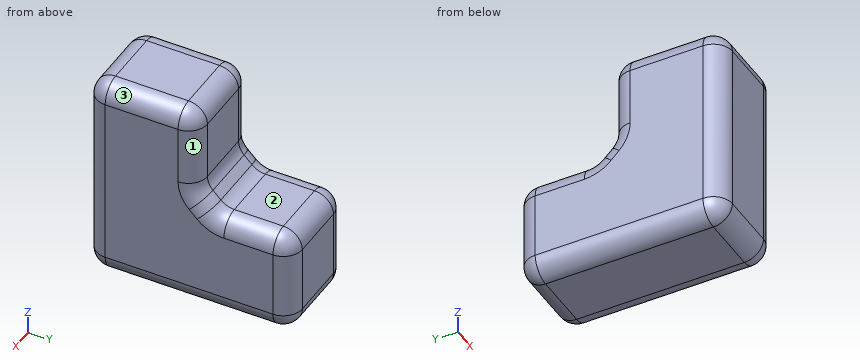
```python
from build123d import *

# Parameters (mm, degrees)
F0_W     = 25.4
F0_H     = 27.94
F1_DEPTH = 25.4
F2_SIZE  = 5.08
F3_F1_R  = 5.08
F3_F2_R  = 5.08


with BuildPart() as f1:
    # F0 (on Right) → F1 (new body)
    with BuildSketch(Plane.YZ):
        Polygon((-14.8341231188, -27.94), (14.8341231188, -27.94), (14.8341231188, 0), (14.8341231188, 27.94), (-14.8341231188, 27.94), align=None)
        with Locations((27.5341231188, -13.97)):
            Rectangle(F0_W, F0_H)
    extrude(amount=F1_DEPTH)

    # F2
    f2_edges = [f1.edges().sort_by_distance(p)[0] for p in [
        (12.7, 14.834123, 0),
    ]]
    chamfer(f2_edges, length=F2_SIZE)

    # F3: fillet of radius 5.08 on 20 edges, made by hand

    # F3_f1
    f3_f1_edges = [f1.edges().sort_by_distance(p)[0] for p in [
        (12.7, 14.8341231188, 5.08),
        (12.7, 19.9141231188, 0),
    ]]
    fillet(f3_f1_edges, radius=F3_F1_R)

    # F3_f2
    f3_f2_edges = [f1.edges().sort_by_distance(p)[0] for p in [
        (12.7, 14.8341231188, 27.94),
        (25.4, 14.8341231188, 17.5621024484),
        (25.4, 0, 27.94),
        (12.7, -14.8341231188, 27.94),
        (0, 0, 27.94),
        (25.4, -14.8341231188, 0),
        (25.4, 12.7, -27.94),
        (25.4, 31.1262255672, 0),
        (25.4, 40.2341231188, -13.97),
        (12.7, 40.2341231188, 0),
        (0, 31.1262255672, 0),
        (0, 40.2341231188, -13.97),
        (12.7, 40.2341231188, -27.94),
        (0, 17.3741231188, 2.54),
        (25.4, 17.3741231188, 2.54),
        (0, 12.7, -27.94),
        (0, -14.8341231188, 0),
        (12.7, -14.8341231188, -27.94),
        (25.4, 20.0742961792, 0.3866919748),
        (25.4, 15.2208150936, 5.2401730604),
        (0, 20.0742961792, 0.3866919748),
        (0, 15.2208150936, 5.2401730604),
    ]]
    fillet(f3_f2_edges, radius=F3_F2_R)


solid = f1.part
```
Here's how the part is built. I have some questions about the finished solid (model axes, mm). Face numbers are marked on the shaded views. A direction names the side the tool comes from. Round coordinates to 2 decimals unless told otherwise and drop trailing zeros. Write each loop counter-clockwise with the first axis right and the second up, starting at its lowest first coordinate (ties: lowest second). Pieces come first, ordered by that corner, then holes.
Q1. If we section it at A-A on y = 1.5: Write out the boundary of the cut face in (x, z).
Q2. Which directions (+Z, -Z, +X, -X, +Y, -Y) give clear straight access to the entire face, cutting with the end or side of a thin tool? Please do the marked faces 1, 2 and 3.
Q3. If we section it at D-D on x = 22.75: Write out the boundary of the cut face in (y, z), plus the area to 3 significant figures.
Q4. Will these pins go through, and if not, where does the flat tip stop? P1, Ø14.5, axis at x = 15, y = 25.5, coming from the +Z side; P2, Ø6, axis at x = 12.5, y = 17, coming from the +Z side; P3, Ø4.5, axis at x = 13.5, z = 12, coming from the +Y side.
Q5. Please list where these lines run through material, in increasing order: probe 1 along Y at (x, z) = (7.5, 22.5); probe 2 along Z at (x, y) = (13, 30); probe 3 along Z at (x, y) = (2.5, 23.5).
Q6. If we section it at B-B on x = 12: Write out the boundary of the cut face in (y, z).
Q7. If we section it at C-C on z = -20.5: Write out the boundary of the cut face in (x, y), plus the area to 3 significant figures.
Answer below:
1. outline: (0, -22.86) arc R5.08 ccw to (5.08, -27.94) - (20.32, -27.94) arc R5.08 ccw to (25.4, -22.86) - (25.4, 22.86) arc R5.08 ccw to (20.32, 27.94) - (5.08, 27.94) arc R5.08 ccw to (0, 22.86) - close
2. face 1: +Z, +X, +Y
2. face 2: +Z, +X, -X, +Y
2. face 3: +Z, +X, +Y, -Y
3. outline: (-14.22, -22.86) arc R4.46 ccw to (-9.75, -27.32) - (35.15, -27.32) arc R4.46 ccw to (39.62, -22.86) - (39.62, -5.08) arc R4.46 ccw to (35.15, -0.62) - (22.02, -0.62) arc R5.7 cw to (17.99, 1.05) - (15.88, 3.15) arc R5.7 cw to (14.22, 7.18) - (14.22, 22.86) arc R4.46 ccw to (9.75, 27.32) - (-9.75, 27.32) arc R4.46 ccw to (-14.22, 22.86) - close
3. area: 2,230 mm2
4. P1: stops at z = 1.66
4. P2: stops at z = 25.65
4. P3: stops at y = 14.83
5. probe 1: y = -14.83 to 14.83
5. probe 2: z = -27.94 to 0
5. probe 3: z = -27.24 to -0.7
6. outline: (-14.83, -22.86) arc R5.08 ccw to (-9.75, -27.94) - (35.15, -27.94) arc R5.08 ccw to (40.23, -22.86) - (40.23, -5.08) arc R5.08 ccw to (35.15, 0) - (22.02, 0) arc R5.08 cw to (18.43, 1.49) - (16.32, 3.59) arc R5.08 cw to (14.83, 7.18) - (14.83, 22.86) arc R5.08 ccw to (9.75, 27.94) - (-9.75, 27.94) arc R5.08 ccw to (-14.83, 22.86) - close
7. outline: (0, -9.75) arc R5.08 ccw to (5.08, -14.83) - (20.32, -14.83) arc R5.08 ccw to (25.4, -9.75) - (25.4, 35.15) arc R5.08 ccw to (20.32, 40.23) - (5.08, 40.23) arc R5.08 ccw to (0, 35.15) - close
7. area: 1,380 mm2
